Can you work these out from the drawing? Everything is in mm from the part's minimum corner. Round coordinates to 2 decimals unless told otherwise and drop trailing zeros. Write each loop counter-clockwise with the first axis right and the second up, starting at its lowest first coordinate (ties: lowest second). Pieces come first, ordered by that corner, then holes. Notation, with made-up numbers: (-28, 56) -> (-20, 56) arc R12 cw to (-20, 65) -> close; hole circle Ø8 at (-31, 63.5). An arc over 180 degrees is marked (long way). Answer as CSV lines item,"result".
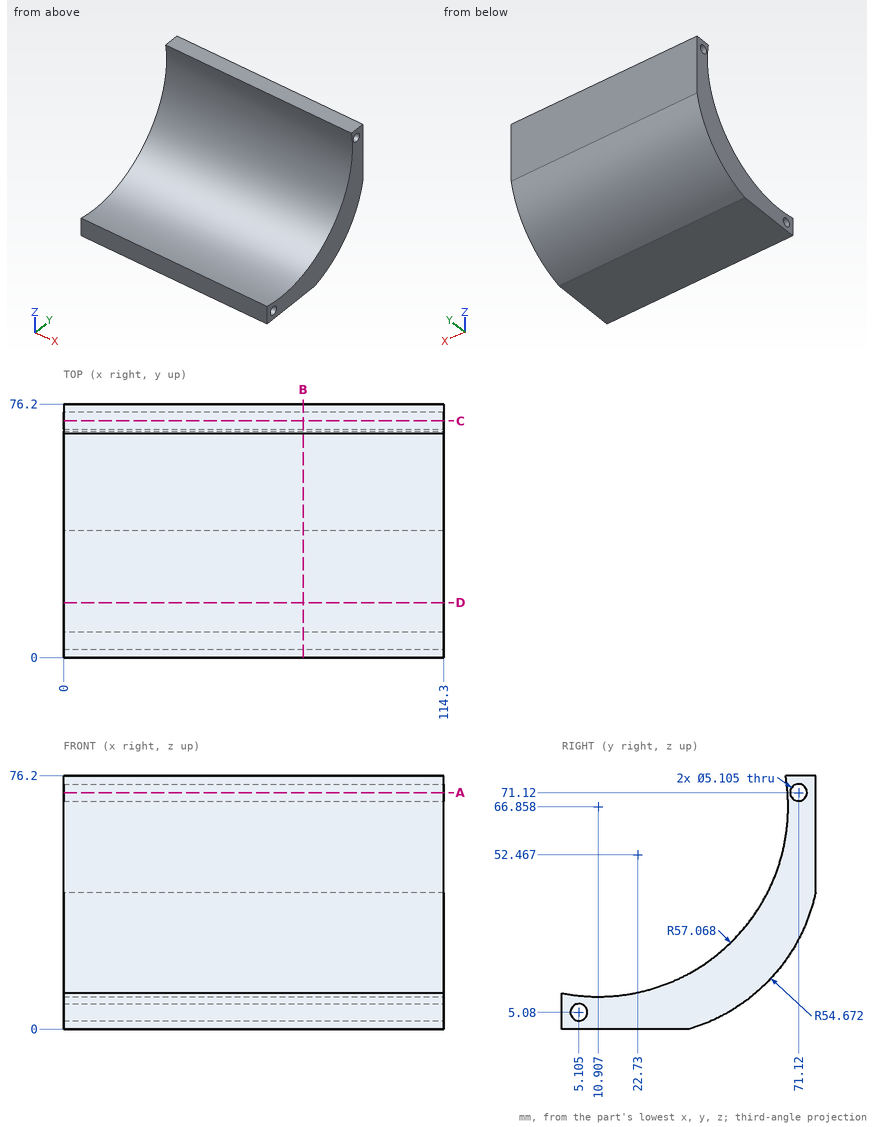
Item 1: Suppose I cut it at D-D, the plane y = 16.5. List the corners of the cut face in (x, z) for me (1 decimal).
Results found:
outline,"(0, 0) -> (114.3, 0) -> (114.3, 10.1) -> (0, 10.1) -> close"
Item 2: I need wall thicknesses on L1, parallel to Y at x = 43, z = 71 (1 decimal); L2, parallel to Y at x = 52.5, z = 4 (1 decimal); L3, parallel to Z at x = 30.5, y = 6. Which ranges of each line are inside material? Lowest first, please.
Results found:
L1,"y = 67.8 to 68.6, 73.7 to 76.2"
L2,"y = 0 to 2.8, 7.4 to 48"
L3,"z = 0 to 2.69, 7.47 to 10"
Item 3: Suppose I cut it at B-B, the plane x = 72. List the corners of the cut face in (y, z) for me (1 decimal).
Results found:
outline,"(0, 0) -> (38.1, 0) arc R54.7 ccw to (76.2, 41.1) -> (76.2, 76.2) -> (67.2, 76.2) arc R57.1 cw to (0, 10.8) -> close; hole circle Ø5.1 at (5.1, 5.1); hole circle Ø5.1 at (71.1, 71.1)"
Item 4: Suppose I cut it at C-C, the plane y = 71.12. List the corners of the cut face in (x, z) for me, then the cut area to 3 significant figures.
Results found:
outline,"(0, 27.02) -> (114.3, 27.02) -> (114.3, 68.57) -> (0, 68.57) -> close; (0, 73.67) -> (114.3, 73.67) -> (114.3, 76.2) -> (0, 76.2) -> close"
area,"5,040 mm²"
Item 5: Will these pins go through, and if not, where does the flat tip stop? pin 1 (10 mm diameter, centred on x = 15.5, z = 39.5, fed in from -Y) (1 decimal); pin 2 (3 mm diameter, centred on x = 30.5, y = 25, fed in from +Z); pin 3 (1 mm diameter, centred on x = 29, z = 26, fed in from +Y).
Results found:
pin 1,"stops at y = 57.9"
pin 2,"stops at z = 11.96"
pin 3,"stops at y = 70.84"
Item 6: Suppose I cut it at A-A, the plane z = 71.12. List the corners of the cut face in (x, y) for me (1 decimal).
Results found:
outline,"(0, 67.8) -> (114.3, 67.8) -> (114.3, 68.6) -> (0, 68.6) -> close; (0, 73.7) -> (114.3, 73.7) -> (114.3, 76.2) -> (0, 76.2) -> close"
